Part model, mm, in its own coordinate system. A direction names the side the tool comes from. Give positions to 0.01 mm unless a question says otherwise; leave off trailing zeros. Write each loop counter-clockwise with the first axis right and the second up, starting at its lowest first coordinate (ties: lowest second). Pieces come first, ordered by that corner, then holes. Notation, with made-up numbers: (73.5, 39.5) - (91.5, 39.5) arc R17 ccw to (91.5, 71.5) - close; hole circle Ø9 at (45, -19). An arc over 180 degrees is marked (long way). Answer in a Markdown table with one row per item. Add a question column.
1. Probe line 1 along Z through (x, y) = (28, 1.65); line 2 along X through (y, z) = (4, -5); line 3 along Z through (x, y) = (58.5, 1.45). List the from-to ranges inside material, lowest first.
2. Which spindle directions (+Z, -Z, +X, -X, +Y, -Y) get a long thin tool onto all of the face, cutting with end or side? Do faces 1 (the flat face through (-1, 2, -90)), 2 (the flat face through (-1, 2, 40)), 3 (the flat face through (52, 2, -40)), 4 (the flat face through (-40, 2, -65)), 5 (the flat face through (0, 2, 0)). Say none if no direction does.
3. Band-saw the part on C-C on x = -6. Write the cut outline in (y, z), plus the area to 3 significant figures.
4. Drop flat-ended pins along their axis: pin 1 Ø5.5 at (x, z) = (43, 8) entering from +Y; pin 2 Ø1.3 at (y, z) = (1, -58.5) entering from +X; pin 3 Ø3 at (x, z) = (57, 8) entering from -Y. Give the stop position or say it passes through.
5. Band-saw the part on D-D on z = 8. Write the cut outline in (x, y).
6. Pull direction X, two halves, no side cores. Call faces 6 (the cylindrical face through (0, 2, -74)), 7 (the flat face through (65, 2, 1)), 8 (the flat face through (-53, 2, -40)): released by +X, released by -X, zero draft, split by the parting line, or undercut.
7. Band-saw the part on A-A on x = -57. Write the cut outline in (y, z).
8. Band-saw the part on B-B on z = 32. Write the cut outline in (x, y), plus the area to 3 significant figures.
```python
from build123d import *

# Parameters (mm, degrees)
SKETCH_2_W          = 130
SKETCH_2_H          = 80
SKETCH_2_R          = 4.9
SKETCH_2_R_2        = 1.65
EXTRUDE_1_DEPTH     = 4.5
SKETCH_3_R          = 2
CUT_EXTRUDE_1_DEPTH = 10
SKETCH_5_W          = 80
SKETCH_5_H          = 50
EXTRUDE_2_DEPTH     = 4.5
SKETCH_6_R          = 4
CUT_EXTRUDE_2_DEPTH = 10
SKETCH_7_R          = 2.25
CUT_EXTRUDE_3_DEPTH = 10
SKETCH_8_R          = 1.25
CUT_EXTRUDE_4_DEPTH = 10
SKETCH_9_W          = 15
SKETCH_9_H          = 60
CUT_EXTRUDE_5_DEPTH = 10
SKETCH_10_R         = 1.25
CUT_EXTRUDE_6_DEPTH = 10


with BuildPart() as part:
    # 草图2 → 凸台-拉伸1 (new body)
    with BuildSketch(Plane(origin=(0, 0, 0), x_dir=(1, 0, 0), z_dir=(0, 1, 0))):
        Rectangle(SKETCH_2_W, SKETCH_2_H)
        with Locations(Location((-50, 0, 0), (0, 0, 270))):
            Circle(SKETCH_2_R, mode=Mode.SUBTRACT)
        with Locations(Location((-57, 8, 0), (0, 0, 270))):
            Circle(SKETCH_2_R_2, mode=Mode.SUBTRACT)
        with Locations(Location((-57, -8, 0), (0, 0, 270))):
            Circle(SKETCH_2_R_2, mode=Mode.SUBTRACT)
        with Locations(Location((-43, 8, 0), (0, 0, 90))):
            Circle(SKETCH_2_R_2, mode=Mode.SUBTRACT)
        with Locations(Location((-43, -8, 0), (0, 0, 90))):
            Circle(SKETCH_2_R_2, mode=Mode.SUBTRACT)
        with Locations(Location((43, 8, 0), (0, 0, 270))):
            Circle(SKETCH_2_R_2, mode=Mode.SUBTRACT)
        with Locations(Location((43, -8, 0), (0, 0, 270))):
            Circle(SKETCH_2_R_2, mode=Mode.SUBTRACT)
        with Locations(Location((57, -8, 0), (0, 0, 90))):
            Circle(SKETCH_2_R_2, mode=Mode.SUBTRACT)
        with Locations(Location((50, 0, 0), (0, 0, 90))):
            Circle(SKETCH_2_R, mode=Mode.SUBTRACT)
        with Locations(Location((57, 8, 0), (0, 0, 90))):
            Circle(SKETCH_2_R_2, mode=Mode.SUBTRACT)
    extrude(amount=EXTRUDE_1_DEPTH)

    # 草图3 → 切除-拉伸1 (cut)
    with BuildSketch(Plane.XZ):
        with Locations(Location((-57, 32, 0), (0, 0, 270))):
            Circle(SKETCH_3_R)
        with Locations(Location((57, 32, 0), (0, 0, 90))):
            Circle(SKETCH_3_R)
        with Locations(Location((57, -32, 0), (0, 0, 270))):
            Circle(SKETCH_3_R)
        with Locations(Location((-57, -32, 0), (0, 0, 90))):
            Circle(SKETCH_3_R)
    extrude(amount=-CUT_EXTRUDE_1_DEPTH, mode=Mode.SUBTRACT)

    # 草图5 → 凸台-拉伸2 (add)
    with BuildSketch(Plane.XZ):
        with Locations((0, -65)):
            Rectangle(SKETCH_5_W, SKETCH_5_H)
    extrude(amount=-EXTRUDE_2_DEPTH)

    # 草图6 → 切除-拉伸2 (cut)
    with BuildSketch(Plane.XZ):
        with Locations(Location((0, -78, 0), (0, 0, 270))):
            Circle(SKETCH_6_R)
    extrude(amount=-CUT_EXTRUDE_2_DEPTH, mode=Mode.SUBTRACT)

    # 草图7 → 切除-拉伸3 (cut)
    with BuildSketch(Plane.XZ):
        with Locations(Location((-14.795139738, 16, 0), (0, 0, 270))):
            Circle(SKETCH_7_R)
        with Locations(Location((14.795139738, 16, 0), (0, 0, 270))):
            Circle(SKETCH_7_R)
    extrude(amount=-CUT_EXTRUDE_3_DEPTH, mode=Mode.SUBTRACT)

    # 草图8 → 切除-拉伸4 (cut)
    with BuildSketch(Plane.XZ):
        with Locations(Location((-28.039056388, -45.101338124, 0), (0, 0, 270))):
            Circle(SKETCH_8_R)
        with Locations(Location((27.968055626, -45.101338124, 0), (0, 0, 270))):
            Circle(SKETCH_8_R)
        with Locations(Location((27.917788926, -86.031350824, 0), (0, 0, 270))):
            Circle(SKETCH_8_R)
        with Locations(Location((-28.039056388, -85.995419912, 0), (0, 0, 270))):
            Circle(SKETCH_8_R)
    extrude(amount=-CUT_EXTRUDE_4_DEPTH, mode=Mode.SUBTRACT)

    # 草图9 → 切除-拉伸5 (cut)
    with BuildSketch(Plane.XZ):
        with Locations((0, -30)):
            Rectangle(SKETCH_9_W, SKETCH_9_H)
    extrude(amount=-CUT_EXTRUDE_5_DEPTH, mode=Mode.SUBTRACT)

    # 草图10 → 切除-拉伸6 (cut)
    with BuildSketch(Plane.XZ):
        with Locations(Location((27.968055626, -9.0699873, 0), (0, 0, 270))):
            Circle(SKETCH_10_R)
        with Locations(Location((-28.039056388, -9.0699873, 0), (0, 0, 270))):
            Circle(SKETCH_10_R)
        with Locations(Location((-28.039056388, -49.964069088, 0), (0, 0, 270))):
            Circle(SKETCH_10_R)
        with Locations(Location((27.917788926, -50, 0), (0, 0, 270))):
            Circle(SKETCH_10_R)
    extrude(amount=-CUT_EXTRUDE_6_DEPTH, mode=Mode.SUBTRACT)


solid = part.part
```
Values:
| question | item | result |
|---|---|---|
| 1 | line 1 | z = -90 to -87.28, -84.78 to -51.25, -48.75 to -46.35, -43.85 to -10.32, -7.82 to 40 |
| 1 | line 2 | x = -65 to -7.5, 7.5 to 65 |
| 1 | line 3 | z = -40 to -33.32, -30.68 to -8.69, -7.31 to 7.31, 8.69 to 30.68, 33.32 to 40 |
| 2 | face 1 | -Z, +X, -X, +Y, -Y |
| 2 | face 2 | +Z, +X, -X, +Y, -Y |
| 2 | face 3 | -Z, +X, +Y, -Y |
| 2 | face 4 | -Z, -X, +Y, -Y |
| 2 | face 5 | +Y, -Y |
| 3 | outline | (0, -90) - (4.5, -90) - (4.5, -60) - (0, -60) - close; (0, 0) - (4.5, 0) - (4.5, 40) - (0, 40) - close |
| 3 | area | 315 mm² |
| 4 | pin 1 | stops at y = 4.5 |
| 4 | pin 2 | stops at x = 40 |
| 4 | pin 3 | passes through |
| 5 | outline | (-65, 0) - (-58.65, 0) - (-58.65, 4.5) - (-65, 4.5) - close; (-55.35, 0) - (-44.65, 0) - (-44.65, 4.5) - (-55.35, 4.5) - close; (-41.35, 0) - (41.35, 0) - (41.35, 4.5) - (-41.35, 4.5) - close; (44.65, 0) - (55.35, 0) - (55.35, 4.5) - (44.65, 4.5) - close; (58.65, 0) - (65, 0) - (65, 4.5) - (58.65, 4.5) - close |
| 6 | face 6 | undercut |
| 6 | face 7 | released by +X |
| 6 | face 8 | zero draft |
| 7 | outline | (0, -40) - (4.5, -40) - (4.5, -34) - (0, -34) - close; (0, -30) - (4.5, -30) - (4.5, -9.65) - (0, -9.65) - close; (0, -6.35) - (4.5, -6.35) - (4.5, 6.35) - (0, 6.35) - close; (0, 9.65) - (4.5, 9.65) - (4.5, 30) - (0, 30) - close; (0, 34) - (4.5, 34) - (4.5, 40) - (0, 40) - close |
| 8 | outline | (-65, 0) - (-59, 0) - (-59, 4.5) - (-65, 4.5) - close; (-55, 0) - (55, 0) - (55, 4.5) - (-55, 4.5) - close; (59, 0) - (65, 0) - (65, 4.5) - (59, 4.5) - close |
| 8 | area | 549 mm² |
